The model under review builds one solid part; all positions refer to its coordinate system, in mm. Give positions to 0.01 mm unless a question says otherwise; leave off trailing zeros. Order: outer loops, then holes, each group sorted by start corner. A loop starts at its lowest first (then second) coordinate and runs counter-clockwise, first axis right, second up. Notation, with made-up numbers: (10, 54) -> (67, 54) arc R29 cw to (67, 74) -> close; hole circle Ø6 at (64.5, -2.5). An arc over 180 degrees is marked (long way). Answer as a JSON object with one key per item and string values. Group by question number.
from build123d import *

# Parameters (mm, degrees)
SKETCH1_W            = 609.6
SKETCH1_H            = 304.8
BOSS_EXTRUDE1_DEPTH  = 3.175
CUT_EXTRUDE1_REACH   = 342.792
FILLET1_R            = 3.175
CUT_EXTRUDE2_REACH   = 342.792
SKETCH4_W            = 38.1
SKETCH4_H            = 38.1
FILLET2_R            = 3.175
FILLET2_OF_MIRROR1_R = 3.175
CUT_EXTRUDE3_REACH   = 342.792
FILLET3_R            = 3.175
FILLET3_OF_MIRROR2_R = 3.175


with BuildPart() as part:
    # Sketch1 → Boss-Extrude1 (new body)
    with BuildSketch(Plane(origin=(0, 0, 0), x_dir=(1, 0, 0), z_dir=(0, 1, 0))):
        Rectangle(SKETCH1_W, SKETCH1_H)
    extrude(amount=BOSS_EXTRUDE1_DEPTH)

    # Sketch3 → Cut-Extrude1 (cut, up to next)
    with BuildSketch(Plane(origin=(0, 3.175, 0), x_dir=(1, 0, 0), z_dir=(0, 1, 0)), mode=Mode.PRIVATE) as cut_extrude1_sk1:
        Polygon((-304.8, 152.4), (304.8, 152.4), (304.8, 57.15), (203.2, 57.15), (203.2, 130.175), (-203.2, 130.175), (-203.2, 57.15), (-304.8, 57.15), align=None)
    cut_extrude1_tool1 = extrude(cut_extrude1_sk1.sketch, amount=-CUT_EXTRUDE1_REACH, mode=Mode.PRIVATE) & part.part
    add(cut_extrude1_tool1.solids().sort_by_distance((0, 3.175, -146.230035))[0], mode=Mode.SUBTRACT)

    # Fillet1
    fillet1_edges = [part.edges().sort_by_distance(p)[0] for p in [
        (203.2, 1.5875, -57.15),
        (-203.2, 1.5875, -57.15),
    ]]
    fillet(fillet1_edges, radius=FILLET1_R)

    # Sketch4 → Cut-Extrude2 (cut, up to next)
    with BuildSketch(Plane(origin=(0, 3.175, 0), x_dir=(1, 0, 0), z_dir=(0, 1, 0)), mode=Mode.PRIVATE) as cut_extrude2_sk1:
        with Locations((239.3315, 38.1)):
            Rectangle(SKETCH4_W, SKETCH4_H)
    cut_extrude2_tool1 = extrude(cut_extrude2_sk1.sketch, amount=-CUT_EXTRUDE2_REACH, mode=Mode.PRIVATE) & part.part
    cut_extrude2 = cut_extrude2_tool1.solids().sort_by_distance((239.3315, 3.175, -38.1))[0]
    add(cut_extrude2, mode=Mode.SUBTRACT)

    # Fillet2
    fillet2_edges = [part.edges().sort_by_distance(p)[0] for p in [
        (258.3815, 1.5875, -19.05),
        (220.2815, 1.5875, -19.05),
    ]]
    fillet(fillet2_edges, radius=FILLET2_R)

    # Mirror1: Cut-Extrude2 across plane
    add(cut_extrude2.mirror(Plane(origin=(0, 0, 0), x_dir=(0, 0, 1), z_dir=(1, 0, 0))), mode=Mode.SUBTRACT)

    # Fillet2 of Mirror1
    fillet2_of_mirror1_edges = [part.edges().sort_by_distance(p)[0] for p in [
        (-258.3815, 1.5875, -19.05),
        (-220.2815, 1.5875, -19.05),
    ]]
    fillet(fillet2_of_mirror1_edges, radius=FILLET2_OF_MIRROR1_R)

    # Sketch5 → Cut-Extrude3 (cut, up to next)
    with BuildSketch(Plane(origin=(0, 3.175, 0), x_dir=(1, 0, 0), z_dir=(0, 1, 0)), mode=Mode.PRIVATE) as cut_extrude3_sk1:
        Polygon((-279.4, -152.4), (-279.4, -124.61875), (-241.3, -124.61875), (-241.3, -118.26875), (-304.8, -118.26875), (-304.8, -152.4), align=None)
    cut_extrude3_tool1 = extrude(cut_extrude3_sk1.sketch, amount=-CUT_EXTRUDE3_REACH, mode=Mode.PRIVATE) & part.part
    cut_extrude3 = cut_extrude3_tool1.solids().sort_by_distance((-285.172727, 3.175, 132.303693))[0]
    add(cut_extrude3, mode=Mode.SUBTRACT)

    # Fillet3
    fillet3_edges = [part.edges().sort_by_distance(p)[0] for p in [
        (-241.3, 1.5875, 124.61875),
        (-241.3, 1.5875, 118.26875),
    ]]
    fillet(fillet3_edges, radius=FILLET3_R - 0.0001)  # a hair under: the kernel refuses the full size

    # Mirror2: Cut-Extrude3 across plane
    add(cut_extrude3.mirror(Plane(origin=(0, 0, 0), x_dir=(0, 0, 1), z_dir=(1, 0, 0))), mode=Mode.SUBTRACT)

    # Fillet3 of Mirror2
    fillet3_of_mirror2_edges = [part.edges().sort_by_distance(p)[0] for p in [
        (241.3, 1.5875, 124.61875),
        (241.3, 1.5875, 118.26875),
    ]]
    fillet(fillet3_of_mirror2_edges, radius=FILLET3_OF_MIRROR2_R - 0.0001)  # a hair under: the kernel refuses the full size


solid = part.part
1. For probe 1 along X at (y, z) = (1.45, -43.5); probe 2 along Z at (x, y) = (-275, 1.6); probe 3 along X at (y, z) = (1.75, -82), list the stretches that pass through material, from the lowest coordinate up. Write a range as [from, to].
2. Take a section at C-C on z = -92.5. Give the boundary of the cut face in (x, y) (3 decimals), plus the area to 3 significant figures.
3. Take a section at A-A on z = -50.5. Give the boundary of the cut face in (x, y) (1 decimal), plus the area to 3 significant figures.
4. For pin 1 (1.6 mm diameter, centred on x = 292, y = 1.5, fed in from -Z); pin 2 (1.6 mm diameter, centred on y = 1, z = -94, fed in from +X); pin 3 (1.6 mm diameter, centred on x = 245, y = 1.5, fed in from -Z), all flat-tipped, find the tip position at first contact; note any pin that passes through.
Checks:
{
 "1": {"probe 1": "x = [-304.8, -258.38], [-220.28, 220.28], [258.38, 304.8]", "probe 2": "z = [-57.15, 118.27], [124.62, 152.4]", "probe 3": "x = [-203.2, 203.2]"},
 "2": {"outline": "(-203.2, 0) -> (203.2, 0) -> (203.2, 3.175) -> (-203.2, 3.175) -> close", "area": "1,290 mm2"},
 "3": {"outline": "(-304.8, 0) -> (-258.4, 0) -> (-258.4, 3.2) -> (-304.8, 3.2) -> close; (-220.3, 0) -> (220.3, 0) -> (220.3, 3.2) -> (-220.3, 3.2) -> close; (258.4, 0) -> (304.8, 0) -> (304.8, 3.2) -> (258.4, 3.2) -> close", "area": "1,690 mm2"},
 "4": {"pin 1": "stops at z = -57.15", "pin 2": "stops at x = 203.2", "pin 3": "stops at z = -19.05"}
}
